```python
from build123d import *

# Parameters (mm, degrees)
SKETCH1_R           = 2
BOSS_EXTRUDE1_DEPTH = 3
SKETCH1_3_W         = 25
SKETCH1_3_H         = 40
BOSS_EXTRUDE4_DEPTH = 3
SKETCH4_W           = 5
SKETCH4_H           = 18
CUT_EXTRUDE1_DEPTH  = 10
SKETCH5_W           = 10
SKETCH5_H           = 18
CUT_EXTRUDE2_DEPTH  = 10
SKETCH8_W           = 10
SKETCH8_H           = 18
CUT_EXTRUDE3_DEPTH  = 10
SKETCH9_W           = 10
SKETCH9_H           = 65
BOSS_EXTRUDE7_DEPTH = 3


with BuildPart() as part:
    # Sketch1 → Boss-Extrude1 (new body)
    with BuildSketch(Plane(origin=(0, 0, 0), x_dir=(1, 0, 0), z_dir=(0, 1, 0))):
        with BuildLine():
            ThreePointArc((-100, 25), (-92.67766953, 7.32233047), (-75, 0))
            Line((-75, 0), (-50, 0))
            Line((-50, 0), (50, 0))
            Line((50, 0), (75, 0))
            ThreePointArc((75, 0), (92.67766953, 7.32233047), (100, 25))
            Line((100, 25), (100, 135))
            Line((100, 135), (90, 135))
            Line((90, 135), (90, 200))
            Line((90, 200), (100, 200))
            Line((100, 200), (100, 220))
            Line((100, 220), (-100, 220))
            Line((-100, 220), (-100, 200))
            Line((-100, 200), (-90, 200))
            Line((-90, 200), (-90, 135))
            Line((-90, 135), (-100, 135))
            Line((-100, 135), (-100, 25))
        make_face()
        with BuildLine():
            Line((-14, 45), (-14, 75))
            ThreePointArc((-14, 75), (-12.5, 76.5), (-11, 75))
            Line((-11, 75), (-11, 45))
            ThreePointArc((-11, 45), (-12.5, 43.5), (-14, 45))
        make_face(mode=Mode.SUBTRACT)
        with BuildLine():
            ThreePointArc((11, 75), (12.5, 76.5), (14, 75))
            Line((14, 75), (14, 45))
            ThreePointArc((14, 45), (12.5, 43.5), (11, 45))
            Line((11, 45), (11, 75))
        make_face(mode=Mode.SUBTRACT)
        with Locations(Location((-90, 110, 0), (0, 0, 270))):
            Circle(SKETCH1_R, mode=Mode.SUBTRACT)
        with Locations(Location((-90, 120, 0), (0, 0, 270))):
            Circle(SKETCH1_R, mode=Mode.SUBTRACT)
        with BuildLine():
            Line((-14, 150), (-14, 180))
            ThreePointArc((-14, 180), (-12.5, 181.5), (-11, 180))
            Line((-11, 180), (-11, 150))
            ThreePointArc((-11, 150), (-12.5, 148.5), (-14, 150))
        make_face(mode=Mode.SUBTRACT)
        with BuildLine():
            Line((-62.5, 211.5), (-12.5, 211.5))
            ThreePointArc((-12.5, 211.5), (-11, 210), (-12.5, 208.5))
            Line((-12.5, 208.5), (-62.5, 208.5))
            ThreePointArc((-62.5, 208.5), (-64, 210), (-62.5, 211.5))
        make_face(mode=Mode.SUBTRACT)
        with Locations(Location((90, 110, 0), (0, 0, 270))):
            Circle(SKETCH1_R, mode=Mode.SUBTRACT)
        with Locations(Location((90, 120, 0), (0, 0, 270))):
            Circle(SKETCH1_R, mode=Mode.SUBTRACT)
        with BuildLine():
            ThreePointArc((11, 180), (12.5, 181.5), (14, 180))
            Line((14, 180), (14, 150))
            ThreePointArc((14, 150), (12.5, 148.5), (11, 150))
            Line((11, 150), (11, 180))
        make_face(mode=Mode.SUBTRACT)
        with BuildLine():
            ThreePointArc((12.5, 208.5), (11, 210), (12.5, 211.5))
            Line((12.5, 211.5), (62.5, 211.5))
            ThreePointArc((62.5, 211.5), (64, 210), (62.5, 208.5))
            Line((62.5, 208.5), (12.5, 208.5))
        make_face(mode=Mode.SUBTRACT)
    extrude(amount=BOSS_EXTRUDE1_DEPTH)

    # Sketch1_3 → Boss-Extrude4 (add)
    with BuildSketch(Plane(origin=(0, 0, 0), x_dir=(1, 0, 0), z_dir=(0, 1, 0))):
        with Locations((-62.5, -20)):
            Rectangle(SKETCH1_3_W, SKETCH1_3_H)
        with Locations((62.5, -20)):
            Rectangle(SKETCH1_3_W, SKETCH1_3_H)
    extrude(amount=BOSS_EXTRUDE4_DEPTH)

    # Sketch4 → Cut-Extrude1 (cut)
    with BuildSketch(Plane(origin=(0, 3, 0), x_dir=(1, 0, 0), z_dir=(0, 1, 0))):
        with Locations((-52.5, -26)):
            Rectangle(SKETCH4_W, SKETCH4_H)
        with Locations((52.5, -26)):
            Rectangle(SKETCH4_W, SKETCH4_H)
    extrude(amount=-CUT_EXTRUDE1_DEPTH, mode=Mode.SUBTRACT)

    # Sketch5 → Cut-Extrude2 (cut)
    with BuildSketch(Plane(origin=(0, 3, 0), x_dir=(1, 0, 0), z_dir=(0, 1, 0))):
        with Locations((60, -26)):
            Rectangle(SKETCH5_W, SKETCH5_H)
    extrude(amount=-CUT_EXTRUDE2_DEPTH, mode=Mode.SUBTRACT)

    # Sketch8 → Cut-Extrude3 (cut)
    with BuildSketch(Plane(origin=(0, 3, 0), x_dir=(1, 0, 0), z_dir=(0, 1, 0))):
        with Locations((-60, -26)):
            Rectangle(SKETCH8_W, SKETCH8_H)
    extrude(amount=-CUT_EXTRUDE3_DEPTH, mode=Mode.SUBTRACT)

    # Sketch9 → Boss-Extrude7 (add)
    with BuildSketch(Plane(origin=(0, 3, 0), x_dir=(1, 0, 0), z_dir=(0, 1, 0))):
        with Locations((-95, 167.5)):
            Rectangle(SKETCH9_W, SKETCH9_H)
        with Locations((95, 167.5)):
            Rectangle(SKETCH9_W, SKETCH9_H)
    extrude(amount=-BOSS_EXTRUDE7_DEPTH)


solid = part.part
```
Source: CAD feature listing. Evaluate the final solid. Frame: model axes, mm. Give positions to 0.01 mm unless a question says otherwise; leave off trailing zeros. Write each loop counter-clockwise with the first axis right and the second up, starting at its lowest first coordinate (ties: lowest second). Pieces come first, ordered by that corner, then holes. Notation, with made-up numbers: (-28.75, 46.5) - (-7.75, 46.5) arc R25 cw to (-7.75, 65.5) - close; hole circle Ø6 at (-33.75, -24.75). An arc over 180 degrees is marked (long way). One line per item, written item: value. Start each with the question number.
Q1. Section query D-D, the plane x = -82. Return the cut outline in (y, z), then the cut area to 3 significant figures.
Q2. Section query C-C, the plane y = 1.6. Count the separate pieces of the cut face and the enclosed holes in it, then the cut area to 3 significant figures.
Q3. First-contact query: pin 1 Ø1.5 at (y, z) = (1.5, 37) entering from +X. Flat tip, straight axial feed; report the tip coordinate or a pass-through.
Q4. Section query A-A, the plane z = 4. Return the cut outline in (x, y).
Q5. Section query B-B, the plane x = 37. Return the cut outline in (y, z).
Q6. Draft query along Y for faces 1 (the face through (92.482, 1.479, -7.129)), 2 (the face through (-1, 0, -92)), 3 (the face through (-1, 3, -92)). Return one class per face: +Y half, -Y half, draft (parallel to the pull), parting line (faces both ways), or undercut.
Q7. Material intervals for probe 1 along Z at (x, y) = (-51, 0.7); probe 2 along X at (y, z) = (1.35, -120); probe 3 along X at (y, z) = (0.2, -51), sorted ascending. Write a range as from..to.
Answer:
1. outline: (0, -220) - (3, -220) - (3, -1) - (0, -1) - close
1. area: 657 mm2
2. separate pieces: 1
2. enclosed holes: 10
2. area: 44,400 mm2
3. pin 1: stops at x = 75
4. outline: (-75, 0) - (-50, 0) - (-50, 3) - (-75, 3) - close; (50, 0) - (75, 0) - (75, 3) - (50, 3) - close
5. outline: (0, -220) - (3, -220) - (3, -211.5) - (0, -211.5) - close; (0, -208.5) - (3, -208.5) - (3, 0) - (0, 0) - close
6. face 1: draft
6. face 2: -Y half
6. face 3: +Y half
7. probe 1: z = -220..-211.5, -208.5..17, 35..40
7. probe 2: x = -100..-92, -88..88, 92..100
7. probe 3: x = -100..-14, -11..11, 14..100
